Geometry check sheet. Reference: the model listing, model coordinates, mm. A direction names the side the tool comes from. Round coordinates to 2 decimals unless told otherwise and drop trailing zeros. Order: outer loops, then holes, each group sorted by start corner. A loop starts at its lowest first (then second) coordinate and runs counter-clockwise, first axis right, second up. Notation, with made-up numbers: (74.25, 86.25) - (121.25, 86.25) arc R19 cw to (121.25, 107.25) - close; hole circle Ø11 at (-36, 23.5). An arc over 180 degrees is marked (long way). Use a Markdown table: item, result. Add a question column.
(1) Access from +Z, -Z, +X, -X, +Y, -Y to the whole of each face (thin tool, end or side, straight path). Record for faces 4 (the face through (0, -4, -122)), 5 (the face through (1.288, 97.251, -128.033)), 6 (the face through (2.54, -2, -122)).
(2) Section check A-A on y = 90. Record the boundary of the cut face in (x, z), then the cut area to 3 significant figures.
(3) Section check C-C on x = 28.5. Record the boundary of the cut face in (y, z).
(4) Section check B-B on z = -155.5. Record the boundary of the cut face in (x, y), then the cut area to 3 significant figures.
(5) Section check D-D on y = 9. Record the boundary of the cut face in (x, z), then the cut area to 3 significant figures.
(6) Thickness scan on line 1 along Y through (x, z) = (26, -100.5); line 2 along X through (y, z) = (2.5, -129). Record the ranges inside material, lowest first. Write a range as [from, to].
(7) Gauge pin test, flat ends, axial feed: P1, Ø4, axis at y = -68.04, z = -119.99, coming from the +X side; P2, Ø10, axis at x = 75.5, z = -98.5, coming from the +Y side; P3, Ø3, axis at y = 75.5, z = -94, coming from the -X side. Record the tip position at first contact, or that the pin passes through.
(8) Mould release check, pull along Y, two halves, no side actions. Record for faces 1 (the face through (51, -121.38, -122)), 2 (the face through (2, -3, -164.449)), 3 (the face through (1.29, 65.44, -111.85)): released by +Y, released by -Y, zero draft, split by the parting line, or undercut.
Autodesk Inventor part; units mm, degrees
ref_plane "YZ Plane" through (0, 0, 0) normal (1, 0, 0) x (0, 1, 0)
ref_plane "XZ Plane" through (0, 0, 0) normal (0, 1, 0) x (-1, 0, 0)
ref_plane "XY Plane" through (0, 0, 0) normal (0, 0, 1) x (1, 0, 0)
sketch "Sketch1" plane through (0, 0, 0) normal (1, 0, 0) x (0, 1, 0)
  line L0 (114.8402, -25.6502) -> (-118.8398, -25.6502)
  line L1 (-118.8398, -25.6502) -> (-118.8398, -330.4502)
  line L2 (-118.8398, -330.4502) -> (114.8402, -330.4502)
  line L3 (114.8402, -330.4502) -> (114.8402, -25.6502)
  point P0 (0, 0)
  dimension "d0" = 233.68
  dimension "d1" = 304.8
extrude "Extrusion1" add sketch "Sketch1" along normal blind 2.54
sketch "Sketch2" plane through (2.54, 0, 0) normal (1, 0, 0) x (0, 0, -1)
  line L0 (25.6502, -118.8398) -> (330.4502, -118.8398)
  line L1 (25.6502, -118.8398) -> (327.6155, -118.8398)
  line L2 (327.6155, -118.8398) -> (327.6155, -121.3798)
  line L3 (327.6155, -121.3798) -> (25.6502, -121.3798)
  line L4 (25.6502, -121.3798) -> (25.6502, -118.8398)
  point P0 (0, 0)
  dimension "d4" = 2.54
extrude "Extrusion2" add sketch "Sketch2" along normal blind 101.6 and the other way blind 2.54
sketch "Sketch3" plane through (2.54, 0, 0) normal (1, 0, 0) x (0, 0, -1)
  line L0 (115.0337, 99.5367) -> (124.9397, 99.5367)
  line L1 (115.0337, 63.0877) -> (124.9397, 63.0877)
  line L2 (108.7599, 94.9012) -> (108.7599, 67.7232)
  line L3 (131.2135, 67.7232) -> (131.2135, 94.9012)
  line L4 (119.9867, 99.5367) -> (119.9867, 63.0877)
  line L5 (119.9867, 81.3122) -> (117.9124, 81.3122)
  line L6 (108.7599, 94.9012) -> (115.0337, 99.5367)
  line L7 (124.9397, 99.5367) -> (131.2135, 94.9012)
  line L8 (108.7599, 67.7232) -> (115.0337, 63.0877)
  line L9 (124.9397, 63.0877) -> (131.2135, 67.7232)
  line L10 (330.4502, 114.8402) -> (25.6502, 114.8402)
  circle A0 centre (108.5567, 111.6652) radius 1.5875
  circle A1 centre (131.4167, 111.6652) radius 1.5875
  circle A2 centre (119.9867, 45.7522) radius 1.5875
  circle A3 centre (119.9867, -11.1438) radius 1.5875
  circle A4 centre (119.9867, -68.0398) radius 1.5875
  circle A5 centre (119.9867, -109.9498) radius 1.5875
  point P0 (0, 0)
  point P1 (108.7599, 81.3122)
  point P2 (119.9867, 63.0877)
  point P3 (131.2135, 81.3122)
  dimension "d9" = 36.449
  dimension "d10" = 22.4536
  dimension "d11" = 11.2268
  dimension "d12" = 9.906
  dimension "d13" = 9.906
  dimension "d14" = 0
  dimension "d15" = 27.178
  dimension "d16" = 27.178
  dimension "d17" = 0
  dimension "d18" = 0
  dimension "d19" = 33.528
  dimension "d20" = 3.175
  dimension "d21" = 3.175
  dimension "d22" = 3.175
  dimension "d23" = 3.175
  dimension "d24" = 11.43
  dimension "d25" = 11.43
  dimension "d26" = 3.175
  dimension "d27" = 3.175
  dimension "d28" = 3.175
  dimension "d29" = 3.175
  dimension "d30" = 0
  dimension "d31" = 0
  dimension "d32" = 0
  dimension "d33" = 69.088
  dimension "d34" = 125.984
  dimension "d35" = 182.88
  dimension "d36" = 224.79
extrude "Extrusion3" cut sketch "Sketch3" against normal blind 101.6
sketch "Sketch4" plane through (0, 114.8402, -25.6502) normal (0, 1, 0) x (1, 0, 0)
  line L0 (0, 304.8) -> (0, 0)
  line L1 (0, 0) -> (2.54, 0)
  line L2 (2.54, 304.8) -> (2.54, 0)
  line L3 (0, 304.8) -> (2.54, 304.8)
  point P0 (0, -25.6502)
extrude "Extrusion4" add sketch "Sketch4" along normal blind 2.54
sketch "Sketch5" plane through (2.54, -118.8398, -25.6502) normal (0, 1, 0) x (1, 0, 0)
  line L0 (-2.54, 0) -> (0, 0)
  line L1 (-2.54, 0) -> (104.5715, 0)
  line L2 (104.5715, 0) -> (104.5715, 52.966)
  line L3 (104.5715, 52.966) -> (-2.54, 52.966)
  line L4 (-2.54, 52.966) -> (-2.54, 0)
  line L5 (101.6, 0) -> (101.6, 301.9653)
  line L6 (-2.54, 304.8) -> (101.6, 304.8)
  line L7 (101.6, 304.8) -> (101.6, 138.7986)
  line L8 (101.6, 138.7986) -> (-2.54, 138.7986)
  line L9 (-2.54, 138.7986) -> (-2.54, 304.8)
  point P0 (-2.54, -25.6502)
  point P1 (101.6, 52.966)
extrude "Extrusion5" cut sketch "Sketch5" along normal through all both and the other way through all contours L4 L3 L5 L1 L0 | L8 L9 L6 L7 L5
properties part number "metal Back for v3.1"
Check sheet entries:
| question | item | result |
|---|---|---|
| 1 | face 4 | +Z, -Z, -X, +Y, -Y |
| 1 | face 5 | +X, -X |
| 1 | face 6 | +Z, -Z, +X, +Y |
| 2 | outline | (0, -164.45) - (2.54, -164.45) - (2.54, -131.21) - (0, -131.21) - close; (0, -108.76) - (2.54, -108.76) - (2.54, -78.62) - (0, -78.62) - close |
| 2 | area | 161 mm2 |
| 3 | outline | (-121.38, -164.45) - (-118.84, -164.45) - (-118.84, -78.62) - (-121.38, -78.62) - close |
| 4 | outline | (0, -121.38) - (104.14, -121.38) - (104.14, -118.84) - (2.54, -118.84) - (2.54, 117.38) - (0, 117.38) - close |
| 4 | area | 865 mm2 |
| 5 | outline | (0, -164.45) - (2.54, -164.45) - (2.54, -78.62) - (0, -78.62) - close |
| 5 | area | 218 mm2 |
| 6 | line 1 | y = [-121.38, -118.84] |
| 6 | line 2 | x = [0, 2.54] |
| 7 | P1 | stops at x = 2.54 |
| 7 | P2 | stops at y = -118.84 |
| 7 | P3 | stops at x = 0 |
| 8 | face 1 | released by -Y |
| 8 | face 2 | zero draft |
| 8 | face 3 | undercut |
